Geometry: final body of the model. Coordinates: model frame, mm. Round coordinates to 2 decimals unless told otherwise and drop trailing zeros. Write each loop counter-clockwise with the first axis right and the second up, starting at its lowest first coordinate (ties: lowest second). Pieces come first, ordered by that corner, then holes. Notation, with made-up numbers: (-34, -3) -> (12, -3) arc R18 ccw to (12, 20) -> close; hole circle Ø7 at (-11.75, 17). An arc over 180 degrees is marked (long way). One line per item, written item: value. Start each with the question number.
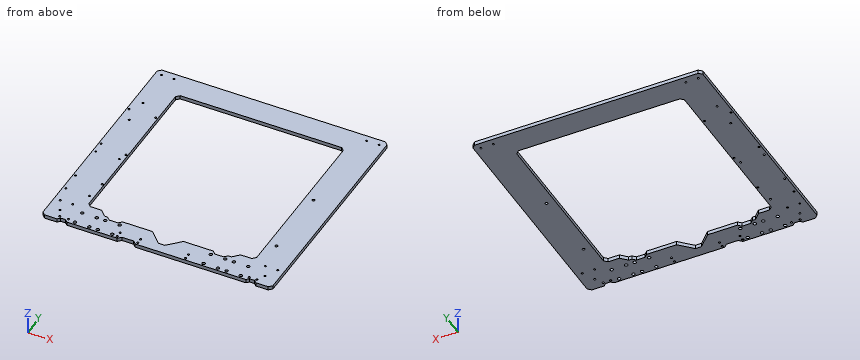
from build123d import *

# Parameters (mm, degrees)
SKICA1_R                = 2.55
SKICA1_R_2              = 1.5
SKICA1_R_3              = 1.6
SKICA1_R_4              = 2.1
P_IDAT_VYSUNUT_M1_DEPTH = 6


with BuildPart() as part:
    # Skica1 → Přidat vysunutím1 (new body)
    with BuildSketch(Plane.XY):
        Polygon((41, 0), (122, 0), (127, 5), (146, 5), (151, 0), (329, 0), (333, 4), (341, 4), (345, 0), (365, 0), (370, 5), (370, 365), (365, 370), (5, 370), (0, 365), (0, 5), (5, 0), (25, 0), (29, 4), (37, 4), align=None)
        with Locations((111.6, 4.9)):
            Circle(SKICA1_R, mode=Mode.SUBTRACT)
        with Locations((111.6, 28.1)):
            Circle(SKICA1_R, mode=Mode.SUBTRACT)
        with Locations((258.4, 28.1)):
            Circle(SKICA1_R, mode=Mode.SUBTRACT)
        with Locations((258.4, 4.9)):
            Circle(SKICA1_R, mode=Mode.SUBTRACT)
        with Locations((88.4, 28.1)):
            Circle(SKICA1_R, mode=Mode.SUBTRACT)
        with Locations((88.4, 4.9)):
            Circle(SKICA1_R, mode=Mode.SUBTRACT)
        with Locations((74.6, 4.9)):
            Circle(SKICA1_R, mode=Mode.SUBTRACT)
        with Locations((74.6, 28.1)):
            Circle(SKICA1_R, mode=Mode.SUBTRACT)
        with Locations((51.4, 28.1)):
            Circle(SKICA1_R, mode=Mode.SUBTRACT)
        with Locations((51.4, 4.9)):
            Circle(SKICA1_R, mode=Mode.SUBTRACT)
        with Locations((281.6, 28.1)):
            Circle(SKICA1_R, mode=Mode.SUBTRACT)
        with Locations((281.6, 4.9)):
            Circle(SKICA1_R, mode=Mode.SUBTRACT)
        with Locations((295.4, 4.9)):
            Circle(SKICA1_R, mode=Mode.SUBTRACT)
        with Locations((318.6, 4.9)):
            Circle(SKICA1_R, mode=Mode.SUBTRACT)
        with Locations((318.6, 28.1)):
            Circle(SKICA1_R, mode=Mode.SUBTRACT)
        with Locations((295.4, 28.1)):
            Circle(SKICA1_R, mode=Mode.SUBTRACT)
        with Locations((3.7, 99.8)):
            Circle(SKICA1_R_2, mode=Mode.SUBTRACT)
        with Locations((47, 99.8)):
            Circle(SKICA1_R_2, mode=Mode.SUBTRACT)
        with Locations((42.9, 67.8)):
            Circle(SKICA1_R_2, mode=Mode.SUBTRACT)
        with Locations((4.9, 67.8)):
            Circle(SKICA1_R_2, mode=Mode.SUBTRACT)
        with Locations((30, 39.8)):
            Circle(SKICA1_R_2, mode=Mode.SUBTRACT)
        with Locations((10, 39.8)):
            Circle(SKICA1_R_2, mode=Mode.SUBTRACT)
        with Locations((20, 19.8)):
            Circle(SKICA1_R_2, mode=Mode.SUBTRACT)
        with Locations((340, 39.8)):
            Circle(SKICA1_R_2, mode=Mode.SUBTRACT)
        with Locations((360, 39.8)):
            Circle(SKICA1_R_2, mode=Mode.SUBTRACT)
        with Locations((340, 359.8)):
            Circle(SKICA1_R_2, mode=Mode.SUBTRACT)
        with Locations((360, 359.8)):
            Circle(SKICA1_R_2, mode=Mode.SUBTRACT)
        with Locations((10, 359.8)):
            Circle(SKICA1_R_2, mode=Mode.SUBTRACT)
        with Locations((30, 359.8)):
            Circle(SKICA1_R_2, mode=Mode.SUBTRACT)
        with Locations((15, 247.8)):
            Circle(SKICA1_R_2, mode=Mode.SUBTRACT)
        with Locations((3.5, 269.3)):
            Circle(SKICA1_R_2, mode=Mode.SUBTRACT)
        with Locations((46.5, 269.3)):
            Circle(SKICA1_R_2, mode=Mode.SUBTRACT)
        with Locations((15, 290.8)):
            Circle(SKICA1_R_2, mode=Mode.SUBTRACT)
        with Locations((4.9, 161.8)):
            Circle(SKICA1_R_2, mode=Mode.SUBTRACT)
        with Locations((3.7, 181.1)):
            Circle(SKICA1_R_2, mode=Mode.SUBTRACT)
        with Locations((42.9, 161.8)):
            Circle(SKICA1_R_2, mode=Mode.SUBTRACT)
        with Locations((47, 174.7)):
            Circle(SKICA1_R_2, mode=Mode.SUBTRACT)
        with Locations((26, 7)):
            Circle(SKICA1_R_3, mode=Mode.SUBTRACT)
        with Locations((40, 7)):
            Circle(SKICA1_R_3, mode=Mode.SUBTRACT)
        with Locations((120, 4)):
            Circle(SKICA1_R_3, mode=Mode.SUBTRACT)
        with Locations((120, 13)):
            Circle(SKICA1_R_3, mode=Mode.SUBTRACT)
        with Locations((153, 13)):
            Circle(SKICA1_R_3, mode=Mode.SUBTRACT)
        with Locations((153, 4)):
            Circle(SKICA1_R_3, mode=Mode.SUBTRACT)
        with Locations((230, 13)):
            Circle(SKICA1_R_3, mode=Mode.SUBTRACT)
        with Locations((230, 4)):
            Circle(SKICA1_R_3, mode=Mode.SUBTRACT)
        with Locations((331, 7)):
            Circle(SKICA1_R_3, mode=Mode.SUBTRACT)
        with Locations((343, 7)):
            Circle(SKICA1_R_3, mode=Mode.SUBTRACT)
        with Locations((350, 19.8)):
            Circle(SKICA1_R_3, mode=Mode.SUBTRACT)
        with Locations((333.4, 88)):
            Circle(SKICA1_R_4, mode=Mode.SUBTRACT)
        with Locations((333.4, 205)):
            Circle(SKICA1_R_4, mode=Mode.SUBTRACT)
        Polygon((320, 51.5), (320, 325), (315, 330), (55, 330), (50, 325), (50, 51.5), (55, 46.5), (73, 46.5), (83, 36.5), (88, 36.5), (93, 31.5), (107, 31.5), (112, 36.5), (160, 36.5), (180, 16.5), (190, 16.5), (210, 36.5), (258, 36.5), (263, 31.5), (277, 31.5), (282, 36.5), (287, 36.5), (297, 46.5), (315, 46.5), align=None, mode=Mode.SUBTRACT)
    extrude(amount=-P_IDAT_VYSUNUT_M1_DEPTH)


solid = part.part
(1) Section query A-A (y = 312.5). Output: boundary loops of the cut face in (x, z), and give its area (3 significant figures).
(2) Line query: probe 1 along Y at (x, z) = (10, -1.25); probe 2 along Y at (x, z) = (130, -2.7); probe 3 along Y at (x, z) = (183, -4.2). Output: solid intervals per line, ascending.
(3) Section query B-B (x = 218). Output: boundary loops of the cut face in (y, z).
(4) Section query C-C (z = -1.6). Count the separate pieces of the cut face and the enclosed holes in it, and give its area (3 significant figures).
(5) Pin query (flat end, axial travel): pin 1 (2.5 mm diameter, centred on x = 3.7, y = 99.8, fed in from +Z). Return the tip coordinate at first contact, or that it passes through.
Results list:
1. outline: (0, -6) -> (50, -6) -> (50, 0) -> (0, 0) -> close; (320, -6) -> (370, -6) -> (370, 0) -> (320, 0) -> close
1. area: 600 mm^2
2. probe 1: y = 0 to 38.3, 41.3 to 358.3, 361.3 to 370
2. probe 2: y = 5 to 36.5, 330 to 370
2. probe 3: y = 0 to 16.5, 330 to 370
3. outline: (0, -6) -> (36.5, -6) -> (36.5, 0) -> (0, 0) -> close; (330, -6) -> (370, -6) -> (370, 0) -> (330, 0) -> close
4. separate pieces: 1
4. enclosed holes: 51
4. area: 56,600 mm^2
5. pin 1: passes through
